Model file for the job. Use its own axes, mm. Face numbers are marked on the shaded views. Round coordinates to 2 decimals unless told otherwise and drop trailing zeros. Loops run counter-clockwise (first coordinate to the right, second up) from the corner with the lowest first, then second, coordinate; pieces in that order, holes last. Notation, with made-up numbers: M 25,76.25 L 81,76.25 A21 ccw 81,83.25 Z; hole C 30,28 d2. An arc over 180 degrees is marked long. Use a Markdown table: item, result. Add a question column.
Q1. Probe line 1 (Y direction, x = 38, z = 10); line 2 (Z direction, x = 84, y = 40.5); line 3 (X direction, y = 14, z = -2.5). List the from-to ranges inside material, lowest first. Write a range as from..to.
Q2. Mould opens along Y. For the marked faces 1, 2 and 3 say: +Y half, -Y half, draft (parallel to the pull), parting line (faces both ways), or undercut.
Q3. Cut at A-A (y = 0). Give the cut face in (x, z).
Q4. Cut at B-B (x = 38.1). Give the cut face in (y, z), plus the area to 3 significant figures.
Q5. Pin check, flat tips, straight feed: pin 1 (1.5 mm diameter, centred on x = 83.5, y = -29, fed in from +Z); pin 2 (1.5 mm diameter, centred on y = -28.5, z = -6, fed in from +X); pin 3 (3 mm diameter, centred on x = 72, z = 0, fed in from +Y). Stop position of each tip, or through.
Q6. Cut at C-C (z = -28.5). Give the cut face in (x, y).
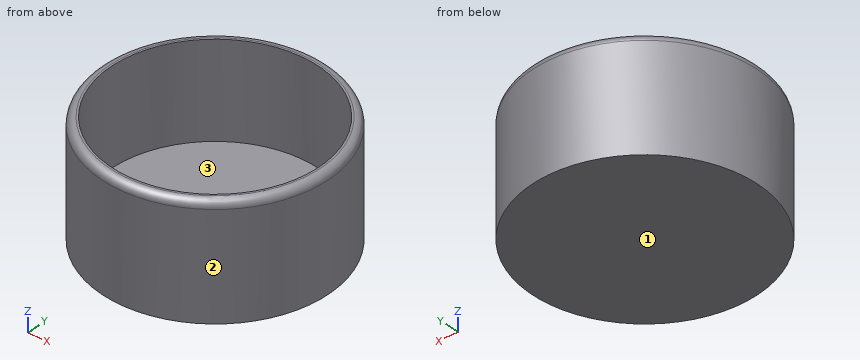
from build123d import *

# Parameters (mm, degrees)
F0_W     = 76.2
F0_H     = 76.2
F2_R     = 69.8500005424
F3_DEPTH = 63.5
F4_R     = 5.08


with BuildPart() as f1:
    # F0 (on Front) → F1 (revolve)
    with BuildSketch(Plane.XZ):
        Rectangle(F0_W, F0_H)
    revolve(axis=Axis((38.1, 0, 0), (0, 0, -1)))

    # F2 (on face) → F3 (cut)
    with BuildSketch(Plane.XY.offset(38.1)):
        with Locations((38.1, 0)):
            Circle(F2_R)
    extrude(amount=-F3_DEPTH, mode=Mode.SUBTRACT)

    # F4
    f4_edges = [f1.edges().sort_by_distance(p)[0] for p in [
        (114.3, 0, 38.1),
    ]]
    fillet(f4_edges, radius=F4_R)


solid = f1.part
Checked values:
| question | item | result |
|---|---|---|
| 1 | line 1 | y = -76.2..-69.85, 69.85..76.2 |
| 1 | line 2 | z = -38.1..-25.4 |
| 1 | line 3 | x = -36.8..-30.33, 106.53..113 |
| 2 | face 1 | draft |
| 2 | face 2 | parting line |
| 2 | face 3 | undercut |
| 3 | outline | M -38.1,-38.1 L 114.3,-38.1 L 114.3,33.02 A5.08 ccw 109.22,38.1 L 107.95,38.1 L 107.95,-25.4 L -31.75,-25.4 L -31.75,38.1 L -33.02,38.1 A5.08 ccw -38.1,33.02 Z |
| 4 | outline | M -76.2,-38.1 L 76.2,-38.1 L 76.2,33.02 A5.08 ccw 71.12,38.1 L 69.85,38.1 L 69.85,-25.4 L -69.85,-25.4 L -69.85,38.1 L -71.12,38.1 A5.08 ccw -76.2,33.02 Z |
| 4 | area | 2,730 mm^2 |
| 5 | pin 1 | stops at z = -25.4 |
| 5 | pin 2 | stops at x = 109.07 |
| 5 | pin 3 | stops at y = 68.97 |
| 6 | outline | C 38.1,0 d152.4 |
